CAD build for the part. Positions are in the model's coordinates, mm. A direction names the side the tool comes from. Coordinates: 2 decimals unless noted, no trailing zeros. Loops run counter-clockwise (first coordinate to the right, second up) from the corner with the lowest first, then second, coordinate; pieces in that order, holes last. Notation, with made-up numbers: (-30, 77) -> (-5, 77) arc R24 cw to (-5, 92) -> close; hole circle Ø6 at (22.5, 82). An arc over 180 degrees is marked (long way). Return JSON: item names as keys, results as strings. Group by question number.
(1) Probe L1, parallel to X at y = -3.65, z = 8.5; L2, parallel to Y at x = 14, z = 3.75; L3, parallel to X at y = -2.5, z = 8. List the from-to ranges inside material, lowest first.
(2) Saw through at D-D on x = 17. Write the cut outline in (y, z).
(3) Saw through at A-A on y = 0. Write the cut outline in (x, z), then the cut area to 3 significant figures.
(4) Saw through at C-C on x = -19. Write the cut outline in (y, z).
(5) Saw through at B-B on z = 2.25. Write the cut outline in (x, y).
(6) Flat gauge pins, fed straight in: pin 1 Ø13 at (x, y) = (0, 0) entering from +Z; pin 2 Ø2.5 at (y, z) = (3.5, 7) entering from +X; pin 3 Ø6.5 at (x, z) = (15.5, 7) entering from +Y; pin 4 Ø1.8 at (x, z) = (14.5, 8.5) entering from +Y. Where does each tip first touch, or does it go through?
(7) Mould opens along X. For faces 4 (the face through (-12.1, -12.81, 11.1)), 5 (the face through (23.846, 7.509, 1.972)), 6 (the face through (-1.85, 22.5, 2.03)) say: pulls with the +X half, pulls with the -X half, needs draft (parallel to the pull), parting line crosses it, or undercut.
(8) Tool access for faces 1 (the face through (-9.03, 7.49, 7.48)), 2 (the face through (17.721, 13.063, 2.028)), 3 (the face through (16, 5.85, 7)): list every direction of +Z, -Z, +X, -X, +Y, -Y with a clear straight run to the whole face (end or side of a thin tool).
```python
from build123d import *

# Parameters (mm, degrees)
SKETCH1_R                = 25
BOSS_EXTRUDE1_DEPTH      = 4
SKETCH2_R                = 5
CUT_EXTRUDE1_DEPTH       = 36.580893749
SKETCH3_W                = 7
SKETCH3_H                = 3.5
BOSS_EXTRUDE2_DEPTH      = 8
FILLET1_R                = 3
SKETCH4_R                = 1.5
CUT_EXTRUDE2_DEPTH       = 42.481592303
FILLET2_R                = 2
CIRPATTERN1_COUNT        = 3
FILLET1_OF_CIRPATTERN1_R = 3
FILLET2_OF_CIRPATTERN1_R = 2
BOSS_EXTRUDE3_START      = 6
SKETCH5_R                = 7
SKETCH5_R_2              = 5
BOSS_EXTRUDE3_DEPTH      = 6
CUT_EXTRUDE3_DEPTH       = 37.249137921
FILLET3_R                = 4
FILLET4_R                = 44
CIRPATTERN2_COUNT        = 3
FILLET3_OF_CIRPATTERN2_R = 4
FILLET4_OF_CIRPATTERN2_R = 44


with BuildPart() as part:
    # Sketch1 → Boss-Extrude1 (new body)
    with BuildSketch(Plane.XY):
        Circle(SKETCH1_R)
    extrude(amount=BOSS_EXTRUDE1_DEPTH)

    # Sketch2 → Cut-Extrude1 (cut, through all)
    with BuildSketch(Plane.XY.offset(4)):
        Circle(SKETCH2_R)
    extrude(amount=-CUT_EXTRUDE1_DEPTH, mode=Mode.SUBTRACT)

    # Sketch3 → Boss-Extrude2 (add)
    with BuildSketch(Plane.XY.offset(4)):
        with Locations((14.5, -4.1)):
            Rectangle(SKETCH3_W, SKETCH3_H)
        with Locations((14.5, 4.1)):
            Rectangle(SKETCH3_W, SKETCH3_H)
    boss_extrude2 = extrude(amount=BOSS_EXTRUDE2_DEPTH)

    # Fillet1
    fillet1_edges = [part.edges().sort_by_distance(p)[0] for p in [
        (11, 4.1, 12),
        (18, 4.1, 12),
        (11, -4.1, 12),
        (18, -4.1, 12),
    ]]
    fillet(fillet1_edges, radius=FILLET1_R)

    # Sketch4 → Cut-Extrude2 (cut, through all)
    with BuildSketch(Plane(origin=(0, 5.85, 0), x_dir=(1, 0, 0), z_dir=(0, 1, 0))):
        with Locations(Location((14.5, -8.5, 0), (0, 0, 270))):
            Circle(SKETCH4_R)
    cut_extrude2 = extrude(amount=-CUT_EXTRUDE2_DEPTH, mode=Mode.SUBTRACT)

    # Fillet2
    fillet2_edges = [part.edges().sort_by_distance(p)[0] for p in [
        (11, 4.1, 4),
        (18, 4.1, 4),
        (11, -4.1, 4),
        (18, -4.1, 4),
    ]]
    fillet(fillet2_edges, radius=FILLET2_R)

    # CirPattern1: Boss-Extrude2, Cut-Extrude2 ×3 about axis
    cirpattern1_axis = Axis((0, 0, 0), (0, 0, 1))
    add([boss_extrude2.rotate(cirpattern1_axis, i * 360 / CIRPATTERN1_COUNT) for i in range(1, CIRPATTERN1_COUNT)])
    add([cut_extrude2.rotate(cirpattern1_axis, i * 360 / CIRPATTERN1_COUNT) for i in range(1, CIRPATTERN1_COUNT)], mode=Mode.SUBTRACT)

    # Fillet1 of CirPattern1
    fillet1_of_cirpattern1_edges = [part.edges().sort_by_distance(p)[0] for p in [
        (-9.050704156, 7.476279442, 12),
        (-12.550704156, 13.538457268, 12),
        (-1.949295844, 11.576279442, 12),
        (-5.449295844, 17.638457268, 12),
        (-1.949295844, -11.576279442, 12),
        (-5.449295844, -17.638457268, 12),
        (-9.050704156, -7.476279442, 12),
        (-12.550704156, -13.538457268, 12),
    ]]
    fillet(fillet1_of_cirpattern1_edges, radius=FILLET1_OF_CIRPATTERN1_R)

    # Fillet2 of CirPattern1
    fillet2_of_cirpattern1_edges = [part.edges().sort_by_distance(p)[0] for p in [
        (-9.050704156, 7.476279442, 4),
        (-12.550704156, 13.538457268, 4),
        (-1.949295844, 11.576279442, 4),
        (-5.449295844, 17.638457268, 4),
        (-1.949295844, -11.576279442, 4),
        (-5.449295844, -17.638457268, 4),
        (-9.050704156, -7.476279442, 4),
        (-12.550704156, -13.538457268, 4),
    ]]
    fillet(fillet2_of_cirpattern1_edges, radius=FILLET2_OF_CIRPATTERN1_R)

    # Sketch5 → Boss-Extrude3 (add)
    with BuildSketch(Plane.XY.offset(4).offset(BOSS_EXTRUDE3_START)):
        Circle(SKETCH5_R)
        Circle(SKETCH5_R_2, mode=Mode.SUBTRACT)
    extrude(amount=-BOSS_EXTRUDE3_DEPTH)

    # Sketch6 → Cut-Extrude3 (cut, through all)
    with BuildSketch(Plane.XY.offset(4)):
        with BuildLine():
            Line((5, 8.660254038), (-2, 20.784609691))
            ThreePointArc((-2, 20.784609691), (-1.833026265, 22.518698234), (-0.139052004, 22.925385473))
            Line((-0.139052004, 22.925385473), (10.706170451, 18.543631176))
            Line((10.706170451, 18.543631176), (19.923492213, 11.342270168))
            ThreePointArc((19.923492213, 11.342270168), (20.418277863, 9.671901806), (19, 8.660254038))
            Line((19, 8.660254038), (5, 8.660254038))
        make_face()
    cut_extrude3 = extrude(amount=-CUT_EXTRUDE3_DEPTH, mode=Mode.SUBTRACT)

    # Fillet3
    fillet3_edges = [part.edges().sort_by_distance(p)[0] for p in [
        (5, 8.660254038, 2),
    ]]
    fillet(fillet3_edges, radius=FILLET3_R)

    # Fillet4
    fillet4_edges = [part.edges().sort_by_distance(p)[0] for p in [
        (10.706170451, 18.543631176, 2),
    ]]
    fillet(fillet4_edges, radius=FILLET4_R)

    # CirPattern2: Cut-Extrude3 ×3 about axis
    cirpattern2_axis = Axis((0, 0, 0), (0, 0, 1))
    for i in range(1, CIRPATTERN2_COUNT):
        add(cut_extrude3.rotate(cirpattern2_axis, i * 360 / CIRPATTERN2_COUNT), mode=Mode.SUBTRACT)

    # Fillet3 of CirPattern2
    fillet3_of_cirpattern2_edges = [part.edges().sort_by_distance(p)[0] for p in [
        (-10, 0, 2),
        (5, -8.660254038, 2),
    ]]
    fillet(fillet3_of_cirpattern2_edges, radius=FILLET3_OF_CIRPATTERN2_R)

    # Fillet4 of CirPattern2
    fillet4_of_cirpattern2_edges = [part.edges().sort_by_distance(p)[0] for p in [
        (-21.412340902, 0, 2),
        (10.706170451, -18.543631176, 2),
    ]]
    fillet(fillet4_of_cirpattern2_edges, radius=FILLET4_OF_CIRPATTERN2_R)


solid = part.part
```
Geometry results:
{
 "1": {"L1": "-5.97 to -3.42, 3.42 to 5.97, 11 to 13, 16 to 18", "L2": "-20.71 to -15.91, -8.66 to 8.66, 15.91 to 20.71", "L3": "-6.54 to -4.33, 4.33 to 6.54, 11 to 13.09, 15.91 to 18"},
 "2": {"outline": "(-18.33, 0) -> (-13.63, 0) -> (-13.63, 4) -> (-18.33, 4) -> close; (-8.66, 0) -> (8.66, 0) -> (8.66, 4) -> (5.85, 4) -> (5.85, 11.24) -> (2.35, 11.24) -> (2.35, 4) -> (-2.35, 4) -> (-2.35, 11.24) -> (-5.85, 11.24) -> (-5.85, 4) -> (-8.66, 4) -> close; (13.63, 0) -> (18.33, 0) -> (18.33, 4) -> (13.63, 4) -> close"},
 "3": {"outline": "(-25, 0) -> (-20.98, 0) -> (-20.98, 4) -> (-25, 4) -> close; (-10.62, 0) -> (-5, 0) -> (-5, 10) -> (-7, 10) -> (-7, 4) -> (-10.62, 4) -> close; (5, 0) -> (25, 0) -> (25, 4) -> (7, 4) -> (7, 10) -> (5, 10) -> close", "area": "143 mm²"},
 "4": {"outline": "(-16.25, 0) -> (-12.7, 0) -> (-12.7, 4) -> (-16.25, 4) -> close; (12.7, 0) -> (16.25, 0) -> (16.25, 4) -> (12.7, 4) -> close"},
 "5": {"outline": "circle Ø50 at (0, 0); hole (-20.55, -6.12) -> (-19.78, -11.58) arc R1.5 ccw to (-17, -12.12) -> (-11.15, -2) arc R4 ccw to (-11.15, 2) -> (-17, 12.12) arc R1.5 ccw to (-19.78, 11.58) -> (-20.55, 6.12) arc R44 ccw to start; hole circle Ø10 at (0, 0); hole (-2, -20.78) arc R1.5 ccw to (-0.14, -22.93) -> (4.97, -20.86) arc R44 ccw to (15.58, -14.74) -> (19.92, -11.34) arc R1.5 ccw to (19, -8.66) -> (7.31, -8.66) arc R4 ccw to (3.85, -10.66) -> close; hole (-2, 20.78) -> (3.85, 10.66) arc R4 ccw to (7.31, 8.66) -> (19, 8.66) arc R1.5 ccw to (19.92, 11.34) -> (15.58, 14.74) arc R44 ccw to (4.97, 20.86) -> (-0.14, 22.93) arc R1.5 ccw to start"},
 "6": {"pin 1": "z = 10", "pin 2": "x = 18.02", "pin 3": "y = 20.54", "pin 4": "through"},
 "7": {"face 4": "pulls with the -X half", "face 5": "parting line crosses it", "face 6": "undercut"},
 "8": {"face 1": "+Z", "face 2": "+Z, -Z", "face 3": "+Z, +X, +Y"}
}
